Source: CAD feature listing. Evaluate the final solid. Frame: model axes, mm. Give positions to 0.01 mm unless a question says otherwise; leave off trailing zeros. Order: outer loops, then holes, each group sorted by start corner. A loop starts at its lowest first (then second) coordinate and runs counter-clockwise, first axis right, second up. Notation, with made-up numbers: (72, -5.75) -> (122, -5.75) arc R36 cw to (122, 33.25) -> close; hole circle Ø5 at (31, 69.25). An arc over 180 degrees is marked (long way). Use one line per item in the form item = value. Start each with the question number.
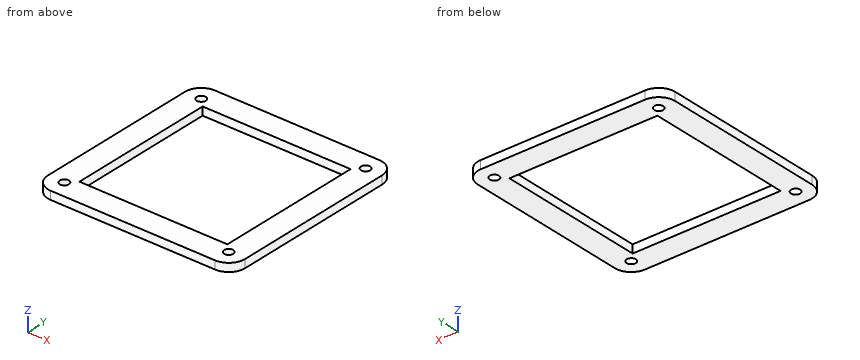
from build123d import *

# Parameters (mm, degrees)
SKETCH1_R           = 2.8
SKETCH1_W           = 90
SKETCH1_H           = 90
BOSS_EXTRUDE1_DEPTH = 5


with BuildPart() as part:
    # Sketch1 → Boss-Extrude1 (new body)
    with BuildSketch(Plane(origin=(0, 0, 0), x_dir=(-1, 0, 0), z_dir=(0, 0, -1))):
        with BuildLine():
            Line((60, -50), (60, 50))
            ThreePointArc((60, 50), (57.071067812, 57.071067812), (50, 60))
            Line((50, 60), (-50, 60))
            ThreePointArc((-50, 60), (-57.071067812, 57.071067812), (-60, 50))
            Line((-60, 50), (-60, -50))
            ThreePointArc((-60, -50), (-57.071067812, -57.071067812), (-50, -60))
            Line((-50, -60), (50, -60))
            ThreePointArc((50, -60), (57.071067812, -57.071067812), (60, -50))
        make_face()
        with Locations(Location((50, -50, 0), (0, 0, 180))):
            Circle(SKETCH1_R, mode=Mode.SUBTRACT)
        with Locations(Location((-50, -50, 0), (0, 0, 180))):
            Circle(SKETCH1_R, mode=Mode.SUBTRACT)
        with Locations(Location((-50, 50, 0), (0, 0, 180))):
            Circle(SKETCH1_R, mode=Mode.SUBTRACT)
        with Locations(Location((50, 50, 0), (0, 0, 180))):
            Circle(SKETCH1_R, mode=Mode.SUBTRACT)
        Rectangle(SKETCH1_W, SKETCH1_H, mode=Mode.SUBTRACT)
    extrude(amount=-BOSS_EXTRUDE1_DEPTH)


solid = part.part
1) Material intervals for probe 1 along Y at (x, z) = (-50, 2.8); probe 2 along X at (y, z) = (-40, 2.2), sorted ascending.
2) Pin query (flat end, axial travel): pin 1 (9 mm diameter, centred on x = -50, y = 50, fed in from +Z). Return the tip coordinate at first contact, or that it passes through.
3) Cut plane C-C, the plane z = 2.9. Return the cut outline in (x, y), plus the area to 3 significant figures.
4) Cut plane A-A, the plane y = 18. Return the cut outline in (x, z), plus the area to 3 significant figures.
Output values:
q1.probe_1 = -60 to -52.8, -47.2 to 47.2, 52.8 to 60
q1.probe_2 = -60 to -45, 45 to 60
q2.pin_1 = 5
q3.outline = (-60, -50) arc R10 ccw to (-50, -60) -> (50, -60) arc R10 ccw to (60, -50) -> (60, 50) arc R10 ccw to (50, 60) -> (-50, 60) arc R10 ccw to (-60, 50) -> close; hole circle Ø5.6 at (-50, -50); hole circle Ø5.6 at (-50, 50); hole (-45, -45) -> (45, -45) -> (45, 45) -> (-45, 45) -> close; hole circle Ø5.6 at (50, -50); hole circle Ø5.6 at (50, 50)
q3.area = 6,120 mm^2
q4.outline = (-60, 0) -> (-45, 0) -> (-45, 5) -> (-60, 5) -> close; (45, 0) -> (60, 0) -> (60, 5) -> (45, 5) -> close
q4.area = 150 mm^2
